from build123d import *

# Parameters (mm, degrees)
F1_DEPTH = 100
F3_DEPTH = 4.001
F4_R     = 5
F5_DEPTH = 4.001
F6_R     = 5
F7_DEPTH = 4.001


# Not quite as in the source:
# - a feature names something its author has since deleted; it is built from what else it names


with BuildPart() as f1:
    # F0 (on Right) → F1 (new body, symmetric)
    with BuildSketch(Plane.YZ):
        with BuildLine():
            Line((0, 192), (0, 0))
            ThreePointArc((0, 0), (-1.1715728753, -2.8284271247), (-4, -4))
            Line((-4, -4), (-46, -4))
            Line((-46, -4), (-46, -8))
            Line((-46, -8), (-4, -8))
            ThreePointArc((-4, -8), (1.6568542495, -5.6568542495), (4, 0))
            Line((4, 0), (4, 192))
            Line((4, 192), (0, 192))
        make_face()
    extrude(amount=F1_DEPTH, both=True)

    # F2 (on face) → F3 (cut, through all)
    with BuildSketch(Plane.XZ):
        with BuildLine():
            Line((-67.5611548883, 152.6005032665), (100, 12))
            Line((100, 12), (100, 192))
            Line((100, 192), (-85, 192))
            ThreePointArc((-85, 192), (-72.3150438383, 185.0057408886), (-71.4596703715, 170.5455849566))
            ThreePointArc((-71.4596703715, 170.5455849566), (-72.5774250894, 160.9067448009), (-67.5611548883, 152.6005032665))
        make_face()
        with BuildLine():
            ThreePointArc((-100, 177), (-95.6066017178, 187.6066017178), (-85, 192))
            Line((-85, 192), (-100, 192))
            Line((-100, 192), (-100, 177))
        make_face()
    extrude(amount=-F3_DEPTH, mode=Mode.SUBTRACT)

    # F4 (on face) → F5 (cut, through all)
    with BuildSketch(Plane.XZ):
        with Locations((-75, 32)):
            Circle(F4_R)
        with Locations((10, 32)):
            Circle(F4_R)
        with Locations((-75, 117)):
            Circle(F4_R)
    extrude(amount=-F5_DEPTH, mode=Mode.SUBTRACT)

    # F6 (on face) → F7 (cut, through all)
    with BuildSketch(Plane.XY.offset(-4)):
        with Locations((-75, -26)):
            Circle(F6_R)
        with Locations((0, -16)):
            Circle(F6_R)
        with Locations((75, -26)):
            Circle(F6_R)
    extrude(amount=-F7_DEPTH, mode=Mode.SUBTRACT)


solid = f1.part
The listing builds one solid part. Answer for the finished solid, in the listing's coordinates (mm). A direction names the side the tool comes from. Give positions to 0.01 mm unless a question says otherwise; leave off trailing zeros. Order: outer loops, then holes, each group sorted by start corner. A loop starts at its lowest first (then second) coordinate and runs counter-clockwise, first axis right, second up. Notation, with made-up numbers: (59.25, 23.25) - (64.25, 23.25) arc R13 cw to (64.25, 39.25) - close; hole circle Ø5 at (15.5, 62). An arc over 180 degrees is marked (long way). One line per item, written item: value. Start each with the question number.
1) A cutting plane is placed at B-B on z = 117. Give the vertices of the cut face in (x, y), then the cut area to 3 significant figures.
2) A cutting plane is placed at C-C on z = 32. Give the vertices of the cut face in (x, y).
3) Find the intervals of material crossed by L1, parallel to Z at x = -75, y = 3.05; L2, parallel to Y at x = 50.5, z = 19.5; L3, parallel to Z at x = 63, y = -34, in increasing order.
4) A cutting plane is placed at A-A on y = -16. Give the vertices of the cut face in (x, z), then the cut area to 3 significant figures.
5) A tool of negligible diameter and unlimited length cuts with its end or side. For faces 1 (the face through (-70.381, -27.915, -5.972)), 2 (the face through (-21, 0, 55)), from which of +Z, -Z, +X, -X, +Y, -Y can it reach the whole face along a straight path? Write none if from no direction.
6) A cutting plane is placed at D-D on x = 10. Give the vertices of the cut face in (y, z), then the cut area to 3 significant figures.
7) The mould has two halves that part along Y. Classify faces 3 (the face through (79.619, -27.915, -5.972)), 4 (the face through (14.619, 1.972, 30.085)), 5 (the face through (1.4, 1.594, -5.719)): released by +Y, released by -Y, zero draft, split by the parting line, or undercut.
8) Given pin 1 Ø12.5 at (x, y) = (25, -17) entering from +Z; pin 2 Ø8 at (x, y) = (-70.5, -2) entering from +Z; pin 3 Ø2 at (x, z) = (31, 20.5) entering from -Y, each flat-ended and moving along its own axis, determine where each tip first touches the part or whether it passes through.
Answer sheet:
1. outline: (-100, 0) - (-80, 0) - (-80, 4) - (-100, 4) - close; (-70, 0) - (-25.13, 0) - (-25.13, 4) - (-70, 4) - close
1. area: 259 mm2
2. outline: (-100, 0) - (-80, 0) - (-80, 4) - (-100, 4) - close; (-70, 0) - (5, 0) - (5, 4) - (-70, 4) - close; (15, 0) - (76.16, 0) - (76.16, 4) - (15, 4) - close
3. L1: z = -3.78 to 27, 37 to 112, 122 to 188.18
3. L2: y = 0 to 4
3. L3: z = -8 to -4
4. outline: (-100, -8) - (-5, -8) - (-5, -4) - (-100, -4) - close; (5, -8) - (100, -8) - (100, -4) - (5, -4) - close
4. area: 760 mm2
5. face 1: +Z, -Z
5. face 2: +Z, +X, -X, -Y
6. outline: (-46, -8) - (-4, -8) arc R8 ccw to (4, 0) - (4, 27) - (0, 27) - (0, 0) arc R4 cw to (-4, -4) - (-46, -4) - close; (0, 37) - (4, 37) - (4, 87.52) - (0, 87.52) - close
6. area: 516 mm2
7. face 3: undercut
7. face 4: zero draft
7. face 5: released by +Y
8. pin 1: stops at z = -4
8. pin 2: stops at z = 187.16
8. pin 3: stops at y = 0
